Could you check a few things on this model? Use its own coordinates, in mm. A direction names the side the tool comes from. Round coordinates to 2 decimals unless told otherwise and drop trailing zeros. Loops run counter-clockwise (first coordinate to the right, second up) from the corner with the lowest first, then second, coordinate; pieces in that order, holes last. Notation, with made-up numbers: (21.5, 57.5) -> (27.5, 57.5) arc R13 ccw to (27.5, 78.5) -> close; hole circle Ø2 at (1, 49). An arc over 180 degrees is marked (long way). One line per item, written item: value.
```python
from build123d import *

# Parameters (mm, degrees)
ESQUISSE1_W                     = 355.6
ESQUISSE1_H                     = 127
BOSS_EXTRU_1_DEPTH              = 6.35
ESQUISSE3_W                     = 25.4
ESQUISSE3_H                     = 6.35
ENL_V_MAT_EXTRU_2_DEPTH         = 6.35
ESQUISSE4_W                     = 6.35
ESQUISSE4_H                     = 12.7
ENL_V_MAT_EXTRU_3_DEPTH         = 25.4
R_P_TITION_LIN_AIRE1_COUNT      = 6
R_P_TITION_LIN_AIRE1_PITCH      = 50.8
R_P_TITION_LIN_AIRE1_COUNT_DIR2 = 2
R_P_TITION_LIN_AIRE1_PITCH_DIR2 = 120.65
R_P_TITION_LIN_AIRE3_COUNT      = 5
R_P_TITION_LIN_AIRE3_PITCH      = 25.4
R_P_TITION_LIN_AIRE3_COUNT_DIR2 = 2
R_P_TITION_LIN_AIRE3_PITCH_DIR2 = 349.25
ESQUISSE5_W                     = 12.7
ESQUISSE5_H                     = 6.35
ENL_V_MAT_EXTRU_4_DEPTH         = 6.35


with BuildPart() as part:
    # Esquisse1 → Boss.-Extru.1 (new body)
    with BuildSketch(Plane(origin=(0, 0, 0), x_dir=(1, 0, 0), z_dir=(0, 1, 0))):
        Rectangle(ESQUISSE1_W, ESQUISSE1_H)
    extrude(amount=BOSS_EXTRU_1_DEPTH)

    # Esquisse3 → Enlèv. mat.-Extru.2 (cut)
    with BuildSketch(Plane(origin=(0, 6.35, 0), x_dir=(1, 0, 0), z_dir=(0, 1, 0))):
        with Locations((-127, 60.325)):
            Rectangle(ESQUISSE3_W, ESQUISSE3_H)
    enl_v_mat_extru_2 = extrude(amount=-ENL_V_MAT_EXTRU_2_DEPTH, mode=Mode.SUBTRACT)

    # Esquisse4 → Enlèv. mat.-Extru.3 (cut)
    with BuildSketch(Plane(origin=(0, 6.35, 0), x_dir=(1, 0, 0), z_dir=(0, 1, 0))):
        with Locations((-174.625, 57.15)):
            Rectangle(ESQUISSE4_W, ESQUISSE4_H)
    enl_v_mat_extru_3 = extrude(amount=-ENL_V_MAT_EXTRU_3_DEPTH, mode=Mode.SUBTRACT)

    # Répétition linéaire1: Enl_v. mat.-Extru.2 6 × 2
    with Locations(*[(i * R_P_TITION_LIN_AIRE1_PITCH, 0, j * R_P_TITION_LIN_AIRE1_PITCH_DIR2) for i in range(R_P_TITION_LIN_AIRE1_COUNT) for j in range(R_P_TITION_LIN_AIRE1_COUNT_DIR2) if (i, j) != (0, 0)]):
        add(enl_v_mat_extru_2, mode=Mode.SUBTRACT)

    # Répétition linéaire3: Enl_v. mat.-Extru.3 5 × 2
    with Locations(*[(j * R_P_TITION_LIN_AIRE3_PITCH_DIR2, 0, i * R_P_TITION_LIN_AIRE3_PITCH) for i in range(R_P_TITION_LIN_AIRE3_COUNT) for j in range(R_P_TITION_LIN_AIRE3_COUNT_DIR2) if (i, j) != (0, 0)]):
        add(enl_v_mat_extru_3, mode=Mode.SUBTRACT)

    # Esquisse5 → Enlèv. mat.-Extru.4 (cut)
    with BuildSketch(Plane(origin=(0, 6.35, 0), x_dir=(1, 0, 0), z_dir=(0, 1, 0))):
        with Locations((-171.45, 60.325)):
            Rectangle(ESQUISSE5_W, ESQUISSE5_H)
        with Locations((171.45, 60.325)):
            Rectangle(ESQUISSE5_W, ESQUISSE5_H)
    extrude(amount=-ENL_V_MAT_EXTRU_4_DEPTH, mode=Mode.SUBTRACT)


solid = part.part
```
(1) On a 3-axis mill with a long thin cutter (end or side, diameter ignored), from which of +Z, -Z, +X, -X, +Y, -Y can I reach the whole of each face in a straight line? I mean faces 1 (the face through (175, 3, -12.7)), 2 (the face through (76, 3, -57.15)), 3 (the face through (-175, 3, -50.8)). Say none if no direction works.
Results below:
face 1: +X, +Y, -Y
face 2: -Z, +Y, -Y
face 3: -Z, -X, +Y, -Y
(2) Imagine slicing it at B-B on x = 83.5. Write out the boundary of the cut face in (y, z), then the cut area to 3 significant figures.
Results below:
outline: (0, -57.15) -> (6.35, -57.15) -> (6.35, 57.15) -> (0, 57.15) -> close
area: 726 mm²
(3) Imagine slicing it at A-A on z = 16.5. Write out the boundary of the cut face in (x, y), then the cut area to 3 significant figures.
Results below:
outline: (-171.45, 0) -> (171.45, 0) -> (171.45, 6.35) -> (-171.45, 6.35) -> close
area: 2,180 mm²
(4) For pin 1 Ø1.5 at (y, z) = (2, 40) entering from +X; pin 2 Ø3 at (y, z) = (2.5, -8) entering from -X; pin 3 Ø1.9 at (y, z) = (3, -59) entering from +X; pin 4 Ø5 at (x, z) = (-117.5, -9.5) entering from -Y, each with a flat end and sliding along its axis, tell me the tip position at first contact or that it passes through.
Results below:
pin 1: stops at x = 171.45
pin 2: stops at x = -171.45
pin 3: stops at x = 165.1
pin 4: stops at y = 0
(5) Please list where these lines run through material, in increasing order: L1, parallel to X at y = 5.75, z = -1.5; L2, parallel to Z at x = 36.5, y = 3.
Results below:
L1: x = -171.45 to 171.45
L2: z = -57.15 to 57.15
(6) We'd pull the mould along X, two halves only. Please class faces 4 (the face through (177.8, 3, 6)), 5 (the face through (-171.45, 3, 19)), 6 (the face through (88.9, 3, 60)): +X half, -X half, draft (parallel to the pull), parting line (faces both ways), or undercut.
Results below:
face 4: +X half
face 5: -X half
face 6: undercut
